Geometry check sheet. Reference: the model listing, model coordinates, mm. A direction names the side the tool comes from. Coordinates: 2 decimals unless noted, no trailing zeros. Order: outer loops, then holes, each group sorted by start corner. A loop starts at its lowest first (then second) coordinate and runs counter-clockwise, first axis right, second up. Notation, with made-up numbers: (87.25, 76.5) -> (114.25, 76.5) arc R8 ccw to (114.25, 90.5) -> close; hole circle Ø7 at (66, 17.25). An arc over 180 degrees is marked (long way). Answer as CSV lines item,"result". Start each with the question number.
from build123d import *

# Parameters (mm, degrees)
SKETCH2_R            = 2.5000000000000004
SKETCH2_R_2          = 2.5000000000000018
BOSS_EXTRUDE1_DEPTH  = 2.5
SKETCH5_W            = 36
SKETCH5_H            = 5
SKETCH11_W           = 51.75
SKETCH11_H           = 51.75
SKETCH11_W_2         = 41.75000000000001
SKETCH11_H_2         = 41.75000000000001
BOSS_EXTRUDE2_DEPTH  = 5
SKETCH14_W           = 41.75000000000001
SKETCH14_H           = 41.75000000000003
BOSS_EXTRUDE3_DEPTH  = 1.5
FILLET1_R            = 8
SKETCH18_R           = 0.8750000000000002
CUT_EXTRUDE3_DEPTH   = 254.3041056928498
CUT_EXTRUDE4_START   = -26.0000001
CUT_EXTRUDE4_DEPTH   = 15.6250001
CUT_EXTRUDE4_START_2 = -2.5
CUT_EXTRUDE4_2_DEPTH = 88.820487138
CUT_EXTRUDE5_DEPTH   = 245.11833407729904
FILLET2_R            = 1.5
BOSS_EXTRUDE4_DEPTH  = 1
FILLET3_R            = 1
SKETCH22_R           = 1.7500000000000062
SKETCH22_R_2         = 1.750000000000084
CUT_EXTRUDE6_DEPTH   = 267.0706428279103
LPATTERN1_COUNT      = 4
LPATTERN1_PITCH      = 40
FILLET4_R            = 5


with BuildPart() as part:
    # Sketch2 → Boss-Extrude1 (new, symmetric)
    with BuildSketch(Plane(origin=(0, 0, 0), x_dir=(1, 0, 0), z_dir=(0, 1, 0))):
        with BuildLine():
            Line((-18.000000000000004, -12.5), (-18, 12.5))
            ThreePointArc((-18, 12.5), (-16.38908729652601, 16.38908729652601), (-12.5, 18.000000000000004))
            Line((-12.5, 18.000000000000004), (12.5, 17.999999999999996))
            Line((12.5, 17.999999999999996), (18.000000000000004, 17.999999999999996))
            Line((18.000000000000004, 17.999999999999996), (18.000000000000004, 12.5))
            Line((18.000000000000004, 12.5), (18.000000000000004, -12.5))
            Line((18.000000000000004, -12.5), (18.000000000000004, -18.000000000000004))
            Line((18.000000000000004, -18.000000000000004), (12.5, -18.000000000000004))
            Line((12.5, -18.000000000000004), (-12.5, -18.000000000000004))
            ThreePointArc((-12.5, -18.000000000000004), (-16.389087296526014, -16.389087296526014), (-18.000000000000004, -12.5))
        make_face()
        with Locations(Location((-12.5, 12.5, 0), (0, 0, 270))):
            Circle(SKETCH2_R, mode=Mode.SUBTRACT)
        with Locations(Location((12.5, 12.5, 0), (0, 0, 270))):
            Circle(SKETCH2_R_2, mode=Mode.SUBTRACT)
        with Locations(Location((12.5, -12.5, 0), (0, 0, 270))):
            Circle(SKETCH2_R_2, mode=Mode.SUBTRACT)
        with Locations(Location((-12.5, -12.5, 0), (0, 0, 270))):
            Circle(SKETCH2_R, mode=Mode.SUBTRACT)
        with Locations(Location((-12.5, 0, 0), (0, 0, 270))):
            Circle(SKETCH2_R, mode=Mode.SUBTRACT)
        with Locations(Location((12.5, 0, 0), (0, 0, 270))):
            Circle(SKETCH2_R, mode=Mode.SUBTRACT)
    extrude(amount=BOSS_EXTRUDE1_DEPTH, both=True)

    # Sweep2: sweep along a path in Sketch4
    with BuildLine(Plane.XY) as sweep2_path:
        Line((218.00000000000003, 97.5), (222.36301639377288, 88.50199533520518))
        ThreePointArc((222.36301639377288, 88.50199533520518), (222.77022201371398, 67.5700619217352), (207.11613369668214, 53.66822133117237))
        Line((207.11613369668214, 53.66822133117237), (25.24812896489628, -1.4262330196007162))
        ThreePointArc((25.24812896489628, -1.4262330196007162), (21.66361669051104, -2.2301013492668282), (18.000000000000004, -2.5))
    # Sketch5 → Sweep2 (sweep)
    with BuildSketch(Plane(origin=(18.000000000000004, 0, 0), x_dir=(0, 0, -1), z_dir=(1, 0, 0))):
        Rectangle(SKETCH5_W, SKETCH5_H)
    sweep(path=sweep2_path.line)

    # Sketch11 → Boss-Extrude2 (add)
    with BuildSketch(Plane(origin=(210.27969021067267, 101.96190931709863, 0), x_dir=(0, 0, 1), z_dir=(-0.8998004664794823, -0.43630163937728456, 0))):
        with Locations((-7.874999999999998, 13.491788097501477)):
            Rectangle(SKETCH11_W, SKETCH11_H)
        with Locations((-7.875000000000001, 13.491788097501482)):
            Rectangle(SKETCH11_W_2, SKETCH11_H_2, mode=Mode.SUBTRACT)
    extrude(amount=-BOSS_EXTRUDE2_DEPTH)

    # Sketch14 → Boss-Extrude3 (add)
    with BuildSketch(Plane(origin=(214.7786925430701, 104.14341751398507, 0), x_dir=(0, 0, -1), z_dir=(0.8998004664794823, 0.43630163937728456, 0))):
        with Locations((7.875000000000001, 13.491788097501479)):
            Rectangle(SKETCH14_W, SKETCH14_H)
    extrude(amount=-BOSS_EXTRUDE3_DEPTH)

    # Fillet1
    fillet1_edges = [part.edges().sort_by_distance(p)[0] for p in [
        (217.93200703068783, 91.91024356915939, -17.999999999999936),
    ]]
    fillet(fillet1_edges, radius=FILLET1_R)

    # Sketch18 → Cut-Extrude3 (cut, through all)
    with BuildSketch(Plane(origin=(210.27969021067267, 101.96190931709863, 0), x_dir=(0, 0, 1), z_dir=(-0.8998004664794823, -0.43630163937728456, 0))):
        with Locations(Location((-7.875000000000007, 36.86678809750149, 0), (0, 0, 270))):
            Circle(SKETCH18_R)
        with Locations(Location((-7.874999999999993, -9.883211902498495, 0), (0, 0, 270))):
            Circle(SKETCH18_R)
    extrude(amount=-CUT_EXTRUDE3_DEPTH, mode=Mode.SUBTRACT)

    # Cut-Extrude4: read off the stored shape, not the designer's step
    # Cut-Extrude4 outline → Cut-Extrude4 (cut)
    with BuildSketch(Plane.XY.offset(CUT_EXTRUDE4_START)):
        with BuildLine():
            ThreePointArc((207.116133697, 53.668221331), (222.268763255, 66.494633739), (223.295688181, 86.320487138))
            Line((223.295688181, 86.320487138), (217.864014061, 86.320487138))
            ThreePointArc((217.864014061, 86.320487138), (218.189778557, 69.574940408), (205.666507904, 58.453467935))
            Line((205.666507904, 58.453467935), (23.798503172, 3.359013584))
            ThreePointArc((23.798503172, 3.359013584), (20.930893352, 2.715918921), (18, 2.5))
            Line((18, 2.5), (-18, 2.5))
            Line((-18, 2.5), (-18, -2.5))
            Line((-18, -2.5), (18, -2.5))
            ThreePointArc((18, -2.5), (21.66361669, -2.230101349), (25.248128965, -1.42623302))
            Line((25.248128965, -1.42623302), (207.116133697, 53.668221331))
        make_face()
    extrude(amount=CUT_EXTRUDE4_DEPTH, mode=Mode.SUBTRACT)

    # Cut-Extrude4 2 outline → Cut-Extrude4 2 (cut)
    with BuildSketch(Plane(origin=(0, 0, 0), x_dir=(1, 0, 0), z_dir=(0, 1, 0)).offset(CUT_EXTRUDE4_START_2)):
        with BuildLine():
            ThreePointArc((-18, 0), (-16.389087297, 3.889087297), (-12.5, 5.5))
            Line((-12.5, 5.5), (196.329521381, 5.5))
            ThreePointArc((196.329521381, 5.5), (201.849371922, 6.116988496), (207.096767721, 7.9375))
            ThreePointArc((207.096767721, 7.9375), (212.34416352, 9.758011504), (217.864014061, 10.375))
            Line((217.864014061, 10.375), (13.816956719, 10.375))
            ThreePointArc((13.816956719, 10.375), (12.5, 10), (11.183043281, 10.375))
            Line((11.183043281, 10.375), (-11.183043281, 10.375))
            ThreePointArc((-11.183043281, 10.375), (-12.5, 10), (-13.816956719, 10.375))
            Line((-13.816956719, 10.375), (-18, 10.375))
            Line((-18, 10.375), (-18, 0))
        make_face()
    extrude(amount=CUT_EXTRUDE4_2_DEPTH, mode=Mode.SUBTRACT)

    # Sketch20 → Cut-Extrude5 (cut, through all)
    with BuildSketch(Plane.XZ.offset(-86.32048713831875)):
        Polygon((223.29568818087398, -10.374999999999993), (193.1038960267146, -10.374999999999996), (193.1038960267146, -33.75), (223.29568818087398, -33.74999999999999), align=None)
    extrude(amount=-CUT_EXTRUDE5_DEPTH, mode=Mode.SUBTRACT)

    # Fillet2
    fillet2_edges = [part.edges().sort_by_distance(p)[0] for p in [
        (215.07564848394176, 96.08201967202383, -10.374999999999993),
        (195.35339719291332, 138.4749177094726, -10.374999999999996),
        (196.86005503994014, 133.64868914754223, -10.374999999999996),
    ]]
    fillet(fillet2_edges, radius=FILLET2_R)

    # Sketch21 → Boss-Extrude4 (add)
    with BuildSketch(Plane.XY.offset(18.000000000000004)):
        with BuildLine():
            Line((-12.5, 2.5), (216.5551091432436, 89.01988853775721))
            Line((216.5551091432436, 89.01988853775721), (217.86401406137549, 86.32048713831875))
            ThreePointArc((217.86401406137549, 86.32048713831875), (218.18977855732837, 69.57494040754278), (205.6665079037029, 58.45346793509252))
            Line((205.6665079037029, 58.45346793509252), (23.79850317191702, 3.3590135843194235))
            ThreePointArc((23.79850317191702, 3.3590135843194235), (20.930893352408834, 2.715918920586539), (18.000000000000004, 2.5))
            Line((18.000000000000004, 2.5), (-12.5, 2.5))
        make_face()
    extrude(amount=-BOSS_EXTRUDE4_DEPTH)

    # Fillet3
    fillet3_edges = [part.edges().sort_by_distance(p)[0] for p in [
        (2.7500000000000018, 2.5, 17.000000000000004),
        (-12.5, 2.5, 17.500000000000004),
        (217.20956160230955, 87.67018783803798, 17.000000000000004),
        (218.18977855732837, 69.57494040754277, 17.000000000000004),
        (114.73250553780996, 30.906240759705973, 17.000000000000004),
        (20.93089335240883, 2.715918920586539, 17.000000000000004),
    ]]
    fillet(fillet3_edges, radius=FILLET3_R)

    # Sketch22 → Cut-Extrude6 (cut, through all)
    with BuildSketch(Plane(origin=(0, 0, 17), x_dir=(-1, 0, 0), z_dir=(0, 0, -1))):
        with Locations((-171.53351288563837, 51.24797304135555)):
            Circle(SKETCH22_R)
        with Locations((-169.79396193406333, 56.99026896605974)):
            Circle(SKETCH22_R_2)
    cut_extrude6 = extrude(amount=-CUT_EXTRUDE6_DEPTH, mode=Mode.SUBTRACT)

    # LPattern1: Cut-Extrude6 ×4
    with Locations(*[Vector(-0.9570493207840286, -0.28992515859585144, 0) * (i * LPATTERN1_PITCH) for i in range(1, LPATTERN1_COUNT)]):
        add(cut_extrude6, mode=Mode.SUBTRACT)

    # Fillet4
    fillet4_edges = [part.edges().sort_by_distance(p)[0] for p in [
        (216.55510914324364, 89.01988853775723, 17.000000000000007),
    ]]
    fillet(fillet4_edges, radius=FILLET4_R)


solid = part.part
Q1. Sectioned sample at B-B, the plane y = 109. Record the cut outline in (x, z) (3 decimals).
Q2. Access from +Z, -Z, +X, -X, +Y, -Y to the whole of each face (thin tool, end or side, straight path). Record for faces 4 (the flat face through (0, 2.5, 6)), 5 (the flat face through (205.31, 112.21, 16.22)), 6 (the cylindrical face through (-16.43, -0.04, -3.85)).
Q3. Thickness scan on L1, parallel to Z at x = 12, y = -1; L2, parallel to Z at x = 51.5, y = 23.5; L3, parallel to X at y = 79, z = 5.5. Record the ranges inside material, lowest first.
Q4. Release check for a two-part mould opening along Z. For faces 1 (the flat face through (130, 47, 17)), 2 (the cylindrical face through (20.97, 2.72, 5.4)), 3 (the cylindrical face through (-14, 0, 10.5)) record: released by +Z, released by -Z, zero draft, split by the parting line, or undercut.
Q5. Sectioned sample at A-A, the plane x = 12.5. Record the cut outline in (y, z).
Q6. Go/stop test with flat-tipped pins: pin 1 Ø6.5 at (x, z) = (-12.5, 12.5) entering from -Y; pin 2 Ø2 at (x, y) = (56.69, 16.46) entering from -Z; pin 3 Ø6 at (y, z) = (92.5, 1.5) entering from -X; pin 4 Ø6 at (x, z) = (71, 0) entering from +Y. Record where each tip stops, or that it passes through.
Geometry results:
1,outline,"(206.867, 13) -> (210.757, 13) -> (210.757, -10.375) -> (212.424, -10.375) -> (212.424, 18) -> (206.867, 18) -> close"
2,face 4,"-Z, -X, +Y"
2,face 5,"-Z, -X"
2,face 6,"-Z, -X, +Y, -Y"
3,L1,"z = -5.5 to -2.45, 2.45 to 10.05, 14.95 to 18"
3,L2,"z = 17 to 18"
3,L3,"x = 219.82 to 224.83"
4,face 1,"released by -Z"
4,face 2,"zero draft"
4,face 3,"undercut"
5,outline,"(-2.5, -5.5) -> (2.5, -5.5) -> (2.5, -2.5) -> (-2.5, -2.5) -> close; (-2.5, 2.5) -> (2.5, 2.5) -> (2.5, 10) -> (-2.5, 10) -> close; (-2.5, 15) -> (2.5, 15) -> (2.5, 16) arc R1 cw to (3.5, 17) -> (11.94, 17) -> (11.94, 18) -> (-2.5, 18) -> close"
6,pin 1,"stops at y = -2.5"
6,pin 2,"passes through"
6,pin 3,"stops at x = 213.5"
6,pin 4,"stops at y = 18.57"
